```python
from build123d import *

# Parameters (mm, degrees)
BOSS_EXTRU_1_DEPTH = 3


with BuildPart() as part:
    # Esquisse1 → Boss.-Extru.1 (new body)
    with BuildSketch(Plane.XY):
        Polygon((-75.988646329, 51.585106383), (-76.753762562, 51.585106383), (-92.861789188, 51.585106383), (-94.860830925, 51.585106383), (-96.789296468, 51.585106383), (-103.253762562, 45.120640289), (-103.253762562, 35.79522772), (-103.253762562, -22.950427523), (-96.789296468, -29.414893617), (63.997857106, -29.414893617), (73.963816863, -26.744522748), (178.515758799, 33.618569072), (237.335031683, 49.379145741), (241.906099495, 57.296467436), (230.508864659, 99.83152691), (225.851857518, 117.211714172), (224.321712805, 123.047343228), (216.426306891, 127.634040432), (210.540810955, 126.057026548), (147.250925797, 109.098552931), (51.669750275, 53.914735514), (42.975455994, 51.585106383), align=None)
        Polygon((-95.09515421, -19.181421764), (-93.057202321, -21.118529255), (-93.715810673, -23.852001108), (-96.412370914, -24.64836547), (-98.450322803, -22.71125798), (-97.791714451, -19.977786126), align=None, mode=Mode.SUBTRACT)
        Polygon((67.767414571, -18.119374886), (69.755583746, -20.107544061), (69.027863321, -22.82343366), (66.311973721, -23.551154085), (64.323804547, -21.56298491), (65.051524972, -18.847095311), align=None, mode=Mode.SUBTRACT)
        Polygon((-93.318762562, 45.490954288), (-93.318762562, 42.679258478), (-95.753762562, 41.273410572), (-98.188762562, 42.679258478), (-98.188762562, 45.490954288), (-95.753762562, 46.896802194), align=None, mode=Mode.SUBTRACT)
        Polygon((-66.988646329, 46.896802194), (-64.553646329, 45.490954288), (-64.553646329, 42.679258478), (-66.988646329, 41.273410572), (-69.423646329, 42.679258478), (-69.423646329, 45.490954288), align=None, mode=Mode.SUBTRACT)
        Polygon((51.366225237, 47.372350111), (51.931744927, 44.618113227), (49.829265662, 42.751240367), (47.161266708, 43.638604392), (46.595747018, 46.392841276), (48.698226283, 48.259714136), align=None, mode=Mode.SUBTRACT)
        Polygon((-76.753762562, 40.085106383), (2.011353671, 40.085106383), (50.71612997, 40.085106383), (151.689760112, 98.382258927), (214.4831558, 115.207698591), (229.494660416, 59.184000666), (174.076924484, 44.334863077), (66.257183131, -17.914893617), (-98.698564415, -17.914893617), (-98.698564415, 40.655573641), (-94.860830925, 40.655573641), (-92.861789188, 40.655573641), (-92.861789188, 48.636078378), (-92.861789188, 50.298812036), (-76.753762562, 50.298812036), (-76.753762562, 49.585106383), (-76.753762562, 48.636078378), align=None, mode=Mode.SUBTRACT)
        Polygon((176.099626255, 43.341034088), (178.27036991, 41.553995947), (177.808121311, 38.780557726), (175.175129056, 37.794157645), (173.004385401, 39.581195786), (173.466634, 42.354634007), align=None, mode=Mode.SUBTRACT)
        Polygon((235.851309069, 58.804459007), (237.257156975, 56.369459007), (235.851309069, 53.934459007), (233.039613258, 53.934459007), (231.633765353, 56.369459007), (233.039613258, 58.804459007), align=None, mode=Mode.SUBTRACT)
        Polygon((150.436891261, 104.94434728), (152.703485209, 103.280560873), (152.395900888, 100.48573973), (149.821722619, 99.354704995), (147.555128671, 101.018491402), (147.862712992, 103.813312544), align=None, mode=Mode.SUBTRACT)
        Polygon((219.824270363, 121.480626406), (219.771686266, 118.66942235), (217.310820089, 117.309359486), (214.90253801, 118.760500678), (214.955122108, 121.571704735), (217.415988284, 122.931767598), align=None, mode=Mode.SUBTRACT)
    extrude(amount=BOSS_EXTRU_1_DEPTH)


solid = part.part
```
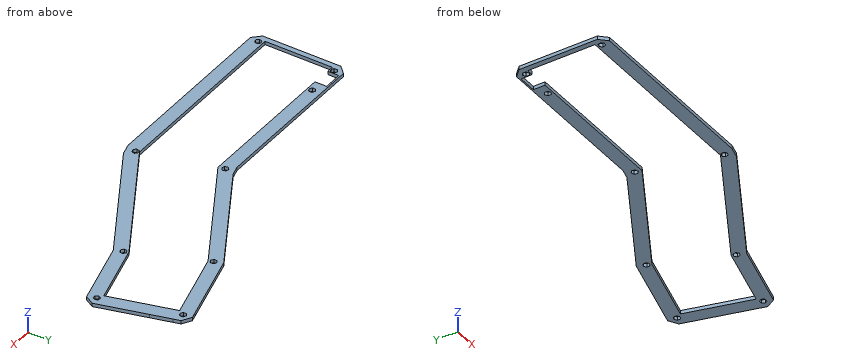
Input: part model. Units: mm. Frame: model coordinates. Give positions to 0.01 mm unless a question says otherwise; leave off trailing zeros. Loops run counter-clockwise (first coordinate to the right, second up) from the corner with the lowest first, then second, coordinate; pieces in that order, holes last.
1) Line query: L1, parallel to Y at x = -55, z = 0.6; L2, parallel to Y at x = -68, z = 2.8; L3, parallel to Y at x = 65.5, z = 2.6. Output: solid intervals per line, ascending.
A:
L1: y = -29.41 to -17.91, 40.09 to 51.59
L2: y = -29.41 to -17.91, 40.09 to 41.86, 46.31 to 51.59
L3: y = -29.01 to -22.74, -18.73 to -17.91, 48.62 to 61.9
2) Section query C-C on z = 0.8. Count the separate pieces of the cut face and the enclosed holes in it, and give its area (3 significant figures).
A:
separate pieces: 1
enclosed holes: 10
area: 8,660 mm2
3) Section query A-A on x = -14. Return the cut outline in (y, z), and give its area (3 significant figures).
A:
outline: (-29.41, 0) - (-17.91, 0) - (-17.91, 3) - (-29.41, 3) - close; (40.09, 0) - (51.59, 0) - (51.59, 3) - (40.09, 3) - close
area: 69.0 mm2
4) Section query B-B on x = 110. Return the cut outline in (y, z).
A:
outline: (-5.94, 0) - (7.34, 0) - (7.34, 3) - (-5.94, 3) - close; (74.31, 0) - (87.59, 0) - (87.59, 3) - (74.31, 3) - close
5) Contact query for flat-ended pins moving along their axis: pin 1 (10 mm diameter, centred on x = 99.5, y = 12, fed in from -Z) (1 decimal); pin 2 (0.9 mm diameter, centred on x = 19.5, z = 2, fed in from +Y); pin 3 (0.8 mm diameter, centred on x = 234, z = 1, fed in from -Y); pin 4 (1.5 mm diameter, centred on y = 10, z = 2, fed in from +X). Output: stop coordinate, or through.
A:
pin 1: passes through
pin 2: stops at y = 51.59
pin 3: stops at y = 48.38
pin 4: stops at x = 138.91
